The listing builds one solid part. Answer for the finished solid, in the listing's coordinates (mm). A direction names the side the tool comes from. Round coordinates to 2 decimals unless told otherwise and drop trailing zeros. Loops run counter-clockwise (first coordinate to the right, second up) from the corner with the lowest first, then second, coordinate; pieces in that order, holes last. Notation, with made-up numbers: (-28.5, 20.25) - (-21.5, 20.25) arc R12 ccw to (-21.5, 36.25) - close; hole circle Ø3 at (-9, 17.25). An arc over 180 degrees is marked (long way). Write item = value, one per line. Start each with the question number.
1) Section C-C, the plane z = -6.5 is taken. Determine the outline of the cut face in (x, y), and give its area (3 significant figures).
2) A tool of negligible diameter and unlimited length cuts with its end or side. For faces 1 (the flat face through (-80, 5, -100)), 2 (the flat face through (-80, 5, 100)), 3 (the flat face through (0, 5, -40)), 4 (the flat face through (123, 5, 100)), from which of +Z, -Z, +X, -X, +Y, -Y can it reach the whole face along a straight path? Write none if from no direction.
3) Straight lines are drawn through the part: line 1 along X through (y, z) = (3, 86); line 2 along X through (y, z) = (0.75, -89.5) (3 decimals); line 3 along Z through (x, y) = (16, 1). For each, find the intervals that lie inside material, in ascending order.
4) Section D-D, the plane y = 4.5 is taken. Give the number of separate pieces and of enclosed holes in the cut face, and give its area (3 significant figures).
5) Given pin 1 Ø1.1 at (x, y) = (88.5, 3.5) entering from +Z; pin 2 Ø1.5 at (x, y) = (88, 6.5) entering from -Z; pin 3 Ø2.5 at (y, z) = (3, 106.5) entering from +X; pin 4 Ø2.5 at (x, z) = (75, -100) entering from +Y, each flat-ended and moving along its own axis, determine where each tip first touches the part or whether it passes through.
6) Section B-B, the plane z = 65 is taken. Determine the outline of the cut face in (x, y), and give its area (3 significant figures).
7) Section A-A, the plane x = 0 is taken. Determine the outline of the cut face in (y, z), and give its area (3 significant figures).
from build123d import *

# Parameters (mm, degrees)
SKETCH1_W            = 260
SKETCH1_H            = 200
EXTRUDE1_DEPTH       = 10
SKETCH3_W            = 20
SKETCH3_H            = 10
EXTRUDE2_DEPTH       = 10
M4_CLEARANCE_HOLE1_D = 4.5
EXTRUDE3_DEPTH       = 10
MIRROR2_COPY_1_DEPTH = 10
MIRROR3_COPY_1_DEPTH = 10
MIRROR3_COPY_2_DEPTH = 10
MIRROR3_COPY_3_DEPTH = 10
SKETCH7_W            = 20
SKETCH7_H            = 10
EXTRUDE4_DEPTH       = 10
LPATTERN1_COUNT      = 2
LPATTERN1_PITCH      = 170
LPATTERN1_COUNT_DIR2 = 2
LPATTERN1_PITCH_DIR2 = 210
EXTRUDE5_DEPTH       = 10
MIRROR5_COPY_1_DEPTH = 10
EXTRUDE6_DEPTH       = 10
MIRROR7_COPY_1_DEPTH = 10
EXTRUDE7_DEPTH       = 10
EXTRUDE8_DEPTH       = 10
M8_CLEARANCE_HOLE1_D = 9


with BuildPart() as part:
    # Sketch1 → Extrude1 (new body)
    with BuildSketch(Plane(origin=(0, 0, 0), x_dir=(1, 0, 0), z_dir=(0, 1, 0))):
        Rectangle(SKETCH1_W, SKETCH1_H)
    extrude(amount=EXTRUDE1_DEPTH)

    # Sketch3 → Extrude2 (cut)
    with BuildSketch(Plane(origin=(0, 10, 0), x_dir=(1, 0, 0), z_dir=(0, 1, 0))):
        with Locations((-105, 45)):
            Rectangle(SKETCH3_W, SKETCH3_H)
        with Locations((105, 45)):
            Rectangle(SKETCH3_W, SKETCH3_H)
        with Locations((-65, 45)):
            Rectangle(SKETCH3_W, SKETCH3_H)
        with Locations((65, 45)):
            Rectangle(SKETCH3_W, SKETCH3_H)
    extrude(amount=-EXTRUDE2_DEPTH, mode=Mode.SUBTRACT)

    # M4 Clearance Hole1 (through all)
    with Locations(Plane(origin=(0, 10, 0), x_dir=(1, 0, 0), z_dir=(0, 1, 0))):
        with Locations((-85, 45), (85, 45)):
            Hole(M4_CLEARANCE_HOLE1_D / 2)

    # Sketch6 → Extrude3 (cut)
    with BuildSketch(Plane(origin=(0, 10, 0), x_dir=(1, 0, 0), z_dir=(0, 1, 0))):
        with BuildLine():
            Line((-113.5, 50), (-115, 50))
            Line((-115, 50), (-115, 48.5))
            ThreePointArc((-115, 48.5), (-116.060660172, 51.060660172), (-113.5, 50))
        make_face()
        with BuildLine():
            Line((-113.5, 40), (-115, 40))
            Line((-115, 40), (-115, 41.5))
            ThreePointArc((-115, 41.5), (-116.060660172, 38.939339828), (-113.5, 40))
        make_face()
    extrude3 = extrude(amount=-EXTRUDE3_DEPTH, mode=Mode.SUBTRACT)

    # Mirror1: Extrude3 across plane
    add(extrude3.mirror(Plane(origin=(-105, 0, 0), x_dir=(0, 0, 1), z_dir=(1, 0, 0))), mode=Mode.SUBTRACT)

    # Mirror2: Extrude3 across plane
    add(extrude3.mirror(Plane.ZY.offset(85)), mode=Mode.SUBTRACT)

    # Mirror2 copy 1 sketch → Mirror2 copy 1 (cut)
    with BuildSketch(Plane(origin=(40, 10, 0), x_dir=(1, 0, 0), z_dir=(0, 1, 0))):
        with BuildLine():
            Line((-113.5, 50), (-115, 50))
            Line((-115, 50), (-115, 48.5))
            ThreePointArc((-115, 48.5), (-116.060660172, 51.060660172), (-113.5, 50))
        make_face()
        with BuildLine():
            Line((-113.5, 40), (-115, 40))
            Line((-115, 40), (-115, 41.5))
            ThreePointArc((-115, 41.5), (-116.060660172, 38.939339828), (-113.5, 40))
        make_face()
    extrude(amount=-MIRROR2_COPY_1_DEPTH, mode=Mode.SUBTRACT)

    # Mirror3: Extrude3 across plane
    add(extrude3.mirror(Plane(origin=(0, 0, 0), x_dir=(0, 0, 1), z_dir=(1, 0, 0))), mode=Mode.SUBTRACT)

    # Mirror3 copy 1 sketch → Mirror3 copy 1 (cut)
    with BuildSketch(Plane(origin=(210, 10, 0), x_dir=(1, 0, 0), z_dir=(0, 1, 0))):
        with BuildLine():
            Line((-113.5, 50), (-115, 50))
            Line((-115, 50), (-115, 48.5))
            ThreePointArc((-115, 48.5), (-116.060660172, 51.060660172), (-113.5, 50))
        make_face()
        with BuildLine():
            Line((-113.5, 40), (-115, 40))
            Line((-115, 40), (-115, 41.5))
            ThreePointArc((-115, 41.5), (-116.060660172, 38.939339828), (-113.5, 40))
        make_face()
    extrude(amount=-MIRROR3_COPY_1_DEPTH, mode=Mode.SUBTRACT)

    # Mirror3 copy 2 sketch → Mirror3 copy 2 (cut)
    with BuildSketch(Plane(origin=(170, 10, 0), x_dir=(1, 0, 0), z_dir=(0, 1, 0))):
        with BuildLine():
            Line((-113.5, 50), (-115, 50))
            Line((-115, 50), (-115, 48.5))
            ThreePointArc((-115, 48.5), (-116.060660172, 51.060660172), (-113.5, 50))
        make_face()
        with BuildLine():
            Line((-113.5, 40), (-115, 40))
            Line((-115, 40), (-115, 41.5))
            ThreePointArc((-115, 41.5), (-116.060660172, 38.939339828), (-113.5, 40))
        make_face()
    extrude(amount=-MIRROR3_COPY_2_DEPTH, mode=Mode.SUBTRACT)

    # Mirror3 copy 3 sketch → Mirror3 copy 3 (cut)
    with BuildSketch(Plane(origin=(-40, 10, 0), x_dir=(-1, 0, 0), z_dir=(0, 1, 0))):
        with BuildLine():
            Line((-113.5, -50), (-115, -50))
            Line((-115, -50), (-115, -48.5))
            ThreePointArc((-115, -48.5), (-116.060660172, -51.060660172), (-113.5, -50))
        make_face()
        with BuildLine():
            Line((-113.5, -40), (-115, -40))
            Line((-115, -40), (-115, -41.5))
            ThreePointArc((-115, -41.5), (-116.060660172, -38.939339828), (-113.5, -40))
        make_face()
    extrude(amount=-MIRROR3_COPY_3_DEPTH, mode=Mode.SUBTRACT)

    # Sketch7 → Extrude4 (add)
    with BuildSketch(Plane(origin=(0, 10, 0), x_dir=(1, 0, 0), z_dir=(0, 1, 0))):
        with Locations((-105, -105)):
            Rectangle(SKETCH7_W, SKETCH7_H)
        with Locations((-65, -105)):
            Rectangle(SKETCH7_W, SKETCH7_H)
    extrude4 = extrude(amount=-EXTRUDE4_DEPTH)

    # LPattern1: Extrude4 2 × 2
    with Locations(*[(i * LPATTERN1_PITCH, 0, -j * LPATTERN1_PITCH_DIR2) for i in range(LPATTERN1_COUNT) for j in range(LPATTERN1_COUNT_DIR2) if (i, j) != (0, 0)]):
        add(extrude4)

    # Sketch8 → Extrude5 (cut)
    with BuildSketch(Plane(origin=(0, 10, 0), x_dir=(1, 0, 0), z_dir=(0, 1, 0))):
        with BuildLine():
            Line((-116.5, -100), (-115, -100))
            Line((-115, -100), (-115, -101.5))
            ThreePointArc((-115, -101.5), (-113.939339828, -98.939339828), (-116.5, -100))
        make_face()
        with BuildLine():
            Line((-95, -101.5), (-95, -100))
            Line((-95, -100), (-93.5, -100))
            ThreePointArc((-93.5, -100), (-96.060660172, -98.939339828), (-95, -101.5))
        make_face()
        with BuildLine():
            Line((-75, -100), (-75, -101.5))
            ThreePointArc((-75, -101.5), (-73.939339828, -98.939339828), (-76.5, -100))
            Line((-76.5, -100), (-75, -100))
        make_face()
        with BuildLine():
            Line((-55, -101.5), (-55, -100))
            Line((-55, -100), (-53.5, -100))
            ThreePointArc((-53.5, -100), (-56.060660172, -98.939339828), (-55, -101.5))
        make_face()
    extrude5 = extrude(amount=-EXTRUDE5_DEPTH, mode=Mode.SUBTRACT)

    # Mirror4: Extrude5 across plane
    add(extrude5.mirror(Plane(origin=(0, 0, 0), x_dir=(0, 0, 1), z_dir=(1, 0, 0))), mode=Mode.SUBTRACT)

    # Mirror5: Extrude5 across plane
    add(extrude5.mirror(Plane.XY), mode=Mode.SUBTRACT)

    # Mirror5 copy 1 sketch → Mirror5 copy 1 (cut)
    with BuildSketch(Plane(origin=(0, 10, 0), x_dir=(-1, 0, 0), z_dir=(0, 1, 0))):
        with BuildLine():
            Line((-116.5, -100), (-115, -100))
            Line((-115, -100), (-115, -101.5))
            ThreePointArc((-115, -101.5), (-113.939339828, -98.939339828), (-116.5, -100))
        make_face()
        with BuildLine():
            Line((-95, -101.5), (-95, -100))
            Line((-95, -100), (-93.5, -100))
            ThreePointArc((-93.5, -100), (-96.060660172, -98.939339828), (-95, -101.5))
        make_face()
        with BuildLine():
            Line((-75, -100), (-75, -101.5))
            ThreePointArc((-75, -101.5), (-73.939339828, -98.939339828), (-76.5, -100))
            Line((-76.5, -100), (-75, -100))
        make_face()
        with BuildLine():
            Line((-55, -101.5), (-55, -100))
            Line((-55, -100), (-53.5, -100))
            ThreePointArc((-53.5, -100), (-56.060660172, -98.939339828), (-55, -101.5))
        make_face()
    extrude(amount=-MIRROR5_COPY_1_DEPTH, mode=Mode.SUBTRACT)

    # Sketch9 → Extrude6 (cut)
    with BuildSketch(Plane(origin=(0, 10, 0), x_dir=(1, 0, 0), z_dir=(0, 1, 0))):
        Polygon((-87.25, -100), (-87.25, -92), (-88.625, -92), (-88.625, -88.3), (-87.25, -88.3), (-87.25, -84), (-82.75, -84), (-82.75, -88.3), (-81.375, -88.3), (-81.375, -92), (-82.75, -92), (-82.75, -100), align=None)
    extrude6 = extrude(amount=-EXTRUDE6_DEPTH, mode=Mode.SUBTRACT)

    # Mirror6: Extrude6 across plane
    add(extrude6.mirror(Plane(origin=(0, 0, 0), x_dir=(0, 0, 1), z_dir=(1, 0, 0))), mode=Mode.SUBTRACT)

    # Mirror7: Extrude6 across plane
    add(extrude6.mirror(Plane.XY), mode=Mode.SUBTRACT)

    # Mirror7 copy 1 sketch → Mirror7 copy 1 (cut)
    with BuildSketch(Plane(origin=(0, 10, 0), x_dir=(-1, 0, 0), z_dir=(0, 1, 0))):
        Polygon((-87.25, -100), (-87.25, -92), (-88.625, -92), (-88.625, -88.3), (-87.25, -88.3), (-87.25, -84), (-82.75, -84), (-82.75, -88.3), (-81.375, -88.3), (-81.375, -92), (-82.75, -92), (-82.75, -100), align=None)
    extrude(amount=-MIRROR7_COPY_1_DEPTH, mode=Mode.SUBTRACT)

    # Sketch10 → Extrude7 (cut)
    with BuildSketch(Plane(origin=(0, 10, 0), x_dir=(1, 0, 0), z_dir=(0, 1, 0))):
        with BuildLine():
            Line((-23, 40), (23, 40))
            Line((23, 40), (23, 18))
            Line((23, 18), (12.5, 18))
            Line((12.5, 18), (12.5, 15.612494996))
            ThreePointArc((12.5, 15.612494996), (0, -20), (-12.5, 15.612494996))
            Line((-12.5, 15.612494996), (-12.5, 18))
            Line((-12.5, 18), (-23, 18))
            Line((-23, 18), (-23, 40))
        make_face()
    extrude(amount=-EXTRUDE7_DEPTH, mode=Mode.SUBTRACT)

    # Sketch11 → Extrude8 (cut)
    with BuildSketch(Plane(origin=(0, 10, 0), x_dir=(1, 0, 0), z_dir=(0, 1, 0))):
        with BuildLine():
            ThreePointArc((53.581713298, -27), (60, 0), (53.581713298, 27))
            ThreePointArc((53.581713298, 27), (40.151427749, 31.43028555), (35.721142199, 18))
            ThreePointArc((35.721142199, 18), (40, 0), (35.721142199, -18))
            ThreePointArc((35.721142199, -18), (40.151427749, -31.43028555), (53.581713298, -27))
        make_face()
        with BuildLine():
            ThreePointArc((-27, -53.581713298), (0, -60), (27, -53.581713298))
            ThreePointArc((27, -53.581713298), (31.43028555, -40.151427749), (18, -35.721142199))
            ThreePointArc((18, -35.721142199), (0, -40), (-18, -35.721142199))
            ThreePointArc((-18, -35.721142199), (-31.43028555, -40.151427749), (-27, -53.581713298))
        make_face()
        with BuildLine():
            ThreePointArc((-53.581713298, 27), (-60, 0), (-53.581713298, -27))
            ThreePointArc((-53.581713298, -27), (-40.151427749, -31.43028555), (-35.721142199, -18))
            ThreePointArc((-35.721142199, -18), (-40, 0), (-35.721142199, 18))
            ThreePointArc((-35.721142199, 18), (-40.151427749, 31.43028555), (-53.581713298, 27))
        make_face()
    extrude(amount=-EXTRUDE8_DEPTH, mode=Mode.SUBTRACT)

    # M8 Clearance Hole1 (through all)
    with Locations(Plane(origin=(0, 10, 0), x_dir=(1, 0, 0), z_dir=(0, 1, 0))):
        with Locations((-65, -65), (65, -65), (65, 65), (-65, 65)):
            Hole(M8_CLEARANCE_HOLE1_D / 2)


solid = part.part
Geometry check:
q1.outline = (-130, 0) - (-59.65, 0) - (-59.65, 10) - (-130, 10) - close; (-39.47, 0) - (-18.91, 0) - (-18.91, 10) - (-39.47, 10) - close; (18.91, 0) - (39.47, 0) - (39.47, 10) - (18.91, 10) - close; (59.65, 0) - (130, 0) - (130, 10) - (59.65, 10) - close
q1.area = 1,820 mm2
q2.face_1 = -Z, +Y, -Y
q2.face_2 = +Z, +Y, -Y
q2.face_3 = +Y, -Y
q2.face_4 = +Z, +X, +Y, -Y
q3.line_1 = -130 to -87.25, -82.75 to 82.75, 87.25 to 130
q3.line_2 = -130 to -88.625, -81.375 to 81.375, 88.625 to 130
q3.line_3 = -100 to -40, -18 to -12, 12 to 36.66, 57.83 to 100
q4.separate_pieces = 1
q4.enclosed_holes = 14
q4.area = 46,000 mm2
q5.pin_1 = 100
q5.pin_2 = -100
q5.pin_3 = 115
q5.pin_4 = through
q6.outline = (-130, 0) - (-69.5, 0) - (-69.5, 10) - (-130, 10) - close; (-60.5, 0) - (60.5, 0) - (60.5, 10) - (-60.5, 10) - close; (69.5, 0) - (130, 0) - (130, 10) - (69.5, 10) - close
q6.area = 2,420 mm2
q7.outline = (0, -100) - (10, -100) - (10, -40) - (0, -40) - close; (0, 20) - (10, 20) - (10, 40) - (0, 40) - close; (0, 60) - (10, 60) - (10, 100) - (0, 100) - close
q7.area = 1,200 mm2
